Drawing for the job (mm, zero at the part's lowest x, y, z). A direction names the side the tool comes from. Coordinates: 2 decimals unless noted, no trailing zeros. Order: outer loops, then holes, each group sorted by start corner. A loop starts at its lowest first (then second) coordinate and runs counter-clockwise, first axis right, second up.
1) Mould opens along Z. For the marked faces 5, 6 and 7 say: +Z half, -Z half, draft (parallel to the pull), parting line (faces both ways), or undercut.
2) Cut at A-A (y = 8). List the corners of the cut face in (x, z).
3) Wall check: L1, parallel to Y at x = 53.25, z = 21; L2, parallel to X at y = 11.25, z = 21; L3, parallel to Z at x = 24, y = 14.25. Give the ranges that are in metal, low to high.
4) Cut at B-B (x = 74). List the corners of the cut face in (y, z), and give its area (3 significant figures).
5) Tool access for the marked faces 1, 2, 3 and 4: list every direction of +Z, -Z, +X, -X, +Y, -Y with a clear straight run to the whole face (end or side of a thin tool).
6) Cut at C-C (z = 21). List the corners of the cut face in (x, y), and give its area (3 significant figures).
7) Cut at D-D (z = 13). List the corners of the cut face in (x, y).
8) Pin check, flat tips, straight feed: pin 1 Ø5 at (y, z) = (19.5, 20) entering from +X; pin 2 Ø12.5 at (x, z) = (28, 30) entering from +Y; pin 3 Ø4 at (x, z) = (67, 34.5) entering from -Y; pin 4 Ø7 at (x, z) = (74, 21) entering from +Y. Stop position of each tip, or through.
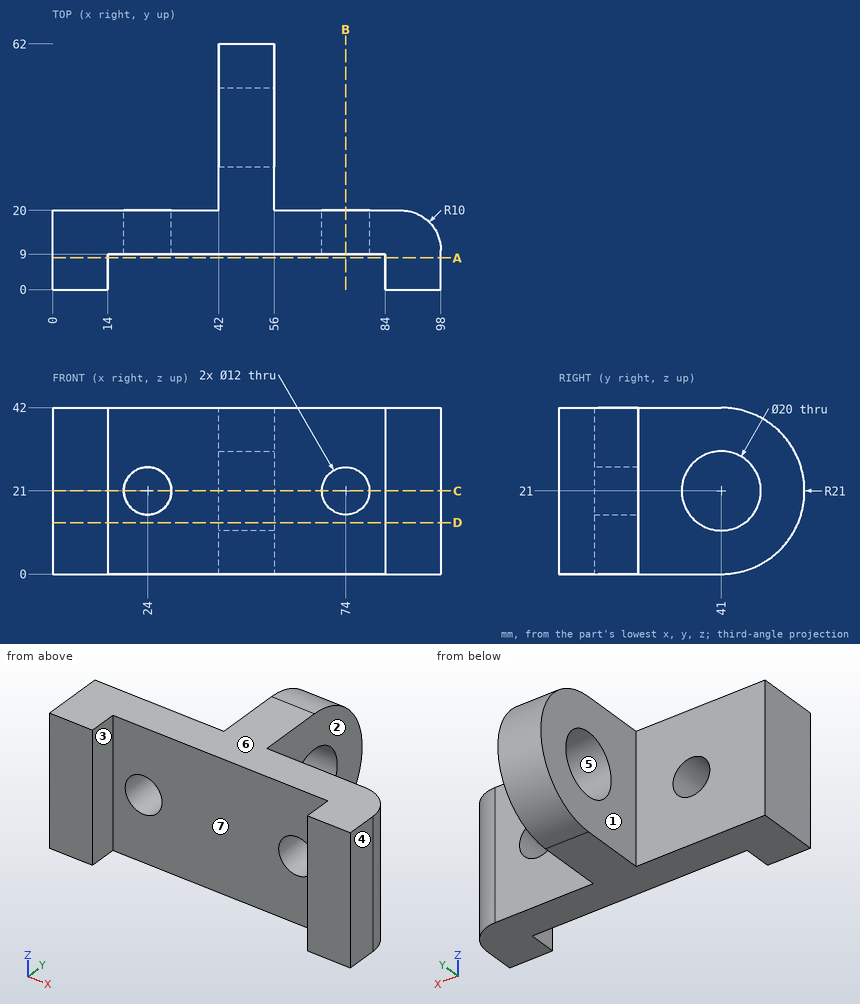
Geometry check:
1. face 5: undercut
1. face 6: +Z half
1. face 7: draft
2. outline: (0, 0) - (14, 0) - (14, 42) - (0, 42) - close; (84, 0) - (98, 0) - (98, 42) - (84, 42) - close
3. L1: y = 9 to 31, 51 to 62
3. L2: x = 0 to 18, 30 to 68, 80 to 97.92
3. L3: z = 0 to 15, 27 to 42
4. outline: (9, 0) - (20, 0) - (20, 15) - (9, 15) - close; (9, 27) - (20, 27) - (20, 42) - (9, 42) - close
4. area: 330 mm2
5. face 1: +Z, -Z, -X, +Y
5. face 2: +Z, -Z, +X, +Y
5. face 3: +Z, -Z, -Y
5. face 4: +Z, -Z, +X, +Y, -Y
6. outline: (0, 0) - (14, 0) - (14, 9) - (18, 9) - (18, 20) - (0, 20) - close; (30, 9) - (68, 9) - (68, 20) - (56, 20) - (56, 31) - (42, 31) - (42, 20) - (30, 20) - close; (42, 51) - (56, 51) - (56, 62) - (42, 62) - close; (80, 9) - (84, 9) - (84, 0) - (98, 0) - (98, 10) arc R10 ccw to (88, 20) - (80, 20) - close
6. area: 1,350 mm2
7. outline: (0, 0) - (14, 0) - (14, 9) - (84, 9) - (84, 0) - (98, 0) - (98, 10) arc R10 ccw to (88, 20) - (56, 20) - (56, 35) - (42, 35) - (42, 20) - (0, 20) - close; (42, 47) - (56, 47) - (56, 60.42) - (42, 60.42) - close
8. pin 1: stops at x = 95.14
8. pin 2: stops at y = 20
8. pin 3: stops at y = 9
8. pin 4: passes through
